from build123d import *

# Parameters (mm, degrees)
F0_W     = 10
F0_H     = 35
F1_DEPTH = 6
F2_W     = 3
F2_H     = 35
F3_DEPTH = 3
F5_DEPTH = 25


with BuildPart() as f1:
    # F0 (on Top) → F1 (new body)
    with BuildSketch(Plane.XY):
        with Locations((5, 17.5)):
            Rectangle(F0_W, F0_H)
    extrude(amount=F1_DEPTH)

    # F2 (on face) → F3 (cut)
    with BuildSketch(Plane.XY.offset(6)):
        with Locations((1.5, 17.5)):
            Rectangle(F2_W, F2_H)
    extrude(amount=-F3_DEPTH, mode=Mode.SUBTRACT)

    # F4 (on face) → F5 (cut)
    with BuildSketch(Plane.XY.offset(6)):
        with BuildLine():
            ThreePointArc((6.5, 23), (7.914214, 23.585786), (8.5, 25))
            ThreePointArc((8.5, 25), (5.085786, 26.414214), (6.5, 23))
        make_face()
    extrude(amount=-F5_DEPTH, mode=Mode.SUBTRACT)


solid = f1.part
Verification items for the finished model (mm, model axes). A direction names the side the tool comes from. Round coordinates to 2 decimals unless told otherwise and drop trailing zeros. Loops run counter-clockwise (first coordinate to the right, second up) from the corner with the lowest first, then second, coordinate; pieces in that order, holes last. Notation, with made-up numbers: (3.5, -37) - (48.5, -37) arc R4 cw to (48.5, -30) - close; hole circle Ø7 at (-8, -40). An arc over 180 degrees is marked (long way). Use a Markdown table: item, result. Add a question column.
1. Section check D-D, the plane z = 5.5. Record the boundary of the cut face in (x, y).
2. Thickness scan on probe 1 along Y at (x, z) = (6.5, 2.85); probe 2 along X at (y, z) = (25, 2.9); probe 3 along Z at (x, y) = (2.5, 11.5). Record the ranges inside material, lowest first. Write a range as [from, to].
3. Section check C-C, the plane y = 15. Record the boundary of the cut face in (x, z), plus the area to 3 significant figures.
4. Access from +Z, -Z, +X, -X, +Y, -Y to the whole of each face (thin tool, end or side, straight path). Record for faces 1 (the face through (0, 17, 1)), 2 (the face through (1, 18, 3)).
5. Section check A-A, the plane x = 5.75. Record the boundary of the cut face in (y, z), plus the area to 3 significant figures.
6. Section check B-B, the plane z = 2.2. Record the boundary of the cut face in (x, y), plus the area to 3 significant figures.
7. Gauge pin test, flat ends, axial feed: pin 1 (1 mm diameter, centred on y = 26.5, z = 4.5, fed in from -X); pin 2 (0.9 mm diameter, centred on x = 2, y = 24, fed in from +Z). Record the tip position at first contact, or that the pin passes through.
Checks:
| question | item | result |
|---|---|---|
| 1 | outline | (3, 0) - (10, 0) - (10, 35) - (3, 35) - close; hole (6.5, 23) arc R2 ccw to (8.5, 25) arc R2 ccw (long way) to start |
| 2 | probe 1 | y = [0, 23], [27, 35] |
| 2 | probe 2 | x = [0, 4.5], [8.5, 10] |
| 2 | probe 3 | z = [0, 3] |
| 3 | outline | (0, 0) - (10, 0) - (10, 6) - (3, 6) - (3, 3) - (0, 3) - close |
| 3 | area | 51.0 mm^2 |
| 4 | face 1 | +Z, -Z, -X, +Y, -Y |
| 4 | face 2 | +Z, -X, +Y, -Y |
| 5 | outline | (0, 0) - (23.15, 0) - (23.15, 6) - (0, 6) - close; (26.85, 0) - (35, 0) - (35, 6) - (26.85, 6) - close |
| 5 | area | 188 mm^2 |
| 6 | outline | (0, 0) - (10, 0) - (10, 35) - (0, 35) - close; hole (6.5, 23) arc R2 ccw to (8.5, 25) arc R2 ccw (long way) to start |
| 6 | area | 337 mm^2 |
| 7 | pin 1 | stops at x = 3 |
| 7 | pin 2 | stops at z = 3 |
